```python
from build123d import *

# Parameters (mm, degrees)
EXTRUDE_1_DEPTH     = 24.5
FILLET_1_R          = 20
FILLET_2_R          = 9
SKETCH_2_W          = 18.5
SKETCH_2_H          = 26.060105981
CUT_EXTRUDE_1_DEPTH = 18
SKETCH_3_W          = 18.5
SKETCH_3_H          = 21.487076152
CUT_EXTRUDE_2_DEPTH = 18
FILLET_3_R          = 1
SKETCH_6_R          = 4
SKETCH_6_R_2        = 3.25
CUT_EXTRUDE_3_DEPTH = 129.841957452
SKETCH_7_R          = 6
CUT_EXTRUDE_4_DEPTH = 10
SKETCH_8_R          = 3.5
CUT_EXTRUDE_5_DEPTH = 127.09619344
EXTRUDE_START       = -10
SKETCH_9_R          = 4
SKETCH_9_R_2        = 3.5
EXTRUDE_2_DEPTH     = 10


with BuildPart() as part:
    # Эскиз1 → Бобышка-Вытянуть1 (new body)
    with BuildSketch(Plane.XY):
        Polygon((0, 0), (0, 40), (120, 40), (120, 0), (100, 0), (100, 29), (20, 29), (20, 0), align=None)
    extrude(amount=EXTRUDE_1_DEPTH)

    # Скругление1
    fillet_1_edges = [part.edges().sort_by_distance(p)[0] for p in [
        (0, 40, 12.25),
        (120, 40, 12.25),
    ]]
    fillet(fillet_1_edges, radius=FILLET_1_R)

    # Скругление2
    fillet_2_edges = [part.edges().sort_by_distance(p)[0] for p in [
        (100, 29, 12.25),
        (20, 29, 12.25),
    ]]
    fillet(fillet_2_edges, radius=FILLET_2_R)

    # Эскиз2 → Вырез-Вытянуть1 (cut)
    with BuildSketch(Plane(origin=(120, 0, 0), x_dir=(0, 0, -1), z_dir=(1, 0, 0))):
        with Locations((-12.25, 33.03005299)):
            Rectangle(SKETCH_2_W, SKETCH_2_H)
    extrude(amount=-CUT_EXTRUDE_1_DEPTH, mode=Mode.SUBTRACT)

    # Эскиз3 → Вырез-Вытянуть2 (cut)
    with BuildSketch(Plane.ZY):
        with Locations((12.25, 30.743538076)):
            Rectangle(SKETCH_3_W, SKETCH_3_H)
    extrude(amount=-CUT_EXTRUDE_2_DEPTH, mode=Mode.SUBTRACT)

    # Скругление3
    fillet_3_edges = [part.edges().sort_by_distance(p)[0] for p in [
        (20, 10, 0),
        (120, 10, 24.5),
        (0, 10, 0),
        (0, 10, 24.5),
        (60, 40, 0),
        (114.142135624, 34.142135624, 0),
        (5.857864376, 34.142135624, 0),
        (60, 40, 24.5),
        (114.142135624, 34.142135624, 24.5),
        (5.857864376, 34.142135624, 24.5),
        (60, 29, 0),
        (60, 29, 24.5),
        (100, 10, 0),
        (100, 10, 24.5),
        (22.636038969, 26.363961031, 0),
        (22.636038969, 26.363961031, 24.5),
        (97.363961031, 26.363961031, 0),
        (97.363961031, 26.363961031, 24.5),
        (20, 10, 24.5),
        (120, 10, 0),
    ]]
    fillet(fillet_3_edges, radius=FILLET_3_R)

    # Эскиз6 → Вырез-Вытянуть3 (cut, through all)
    with BuildSketch(Plane(origin=(0, 0, 0), x_dir=(-1, 0, 0), z_dir=(0, -1, 0))):
        with Locations(Location((-10, -12.25, 0), (0, 0, 180))):
            Circle(SKETCH_6_R)
        with Locations(Location((-110, -12.25, 0), (0, 0, 180))):
            Circle(SKETCH_6_R_2)
    extrude(amount=-CUT_EXTRUDE_3_DEPTH, mode=Mode.SUBTRACT)

    # Эскиз7 → Вырез-Вытянуть4 (cut)
    with BuildSketch(Plane(origin=(0, 20, 0), x_dir=(1, 0, 0), z_dir=(0, 1, 0))):
        with Locations(Location((10, -12.25, 0), (0, 0, 270))):
            Circle(SKETCH_7_R)
        with Locations(Location((110, -12.25, 0), (0, 0, 270))):
            Circle(SKETCH_7_R)
    extrude(amount=-CUT_EXTRUDE_4_DEPTH, mode=Mode.SUBTRACT)

    # Эскиз8 → Вырез-Вытянуть5 (cut, through all)
    with BuildSketch(Plane(origin=(0, 10, 0), x_dir=(1, 0, 0), z_dir=(0, 1, 0))):
        with Locations(Location((110, -12.25, 0), (0, 0, 270))):
            Circle(SKETCH_8_R)
    extrude(amount=-CUT_EXTRUDE_5_DEPTH, mode=Mode.SUBTRACT)

    # Эскиз9 → Бобышка-Вытянуть2 (add)
    with BuildSketch(Plane(origin=(0, 10, 0), x_dir=(1, 0, 0), z_dir=(0, 1, 0)).offset(EXTRUDE_START)):
        with Locations((10, -12.25)):
            Circle(SKETCH_9_R)
        with Locations(Location((10, -12.25, 0), (0, 0, 270))):
            Circle(SKETCH_9_R_2, mode=Mode.SUBTRACT)
    extrude(amount=EXTRUDE_2_DEPTH)


solid = part.part
```
For this review, take the finished solid that the model builds, in its own axes (mm). A direction names the side the tool comes from. Coordinates: 2 decimals unless noted, no trailing zeros. Loops run counter-clockwise (first coordinate to the right, second up) from the corner with the lowest first, then second, coordinate; pieces in that order, holes last. Notation, with made-up numbers: (69.5, 59.5) - (123.5, 59.5) arc R19 ccw to (123.5, 76.5) - close; hole circle Ø3 at (49, 82). An arc over 180 degrees is marked (long way). Use one line per item in the form item = value. Start each with the question number.
1) For faces 1 (the face through (112, 0, 9)), 2 (the face through (22.566, 26.294, 12.408)), 3 (the face through (11, 28, 21.5)), 4 (the face through (4.677, 15.07, 15.019)), 5 (the face through (6.583, 4.93, 11.491)), list the 3-axis set-ups (+Z, -Z, +X, -X, +Y, -Y) from which the entire face can be reached by the end or side of a thin tool; tool diameter is ignored.
2) Take a section at A-A (z = 12.25). State how many separate pieces and enclosed holes the cut face has, plus the area to 3 significant figures.
3) Draft analysis for pull direction X (two halves, no side actions). For faces 6 (the face through (13, 10, 15)), 7 (the face through (115, 20, 16)), 8 (the face through (18.184, 39.917, 10.636)), state which applies: released by +X, released by -X, zero draft, split by the parting line, or undercut.
4) Take a section at C-C (z = 7.5). State the section outline as (x, y) points, plus the area to 3 significant figures.
5) To check wall thickness, follow probe 1 along X at (y, z) = (15.5, 12.25); probe 2 along X at (y, z) = (2.5, 12.25); probe 3 along Z at (x, y) = (106, 21). State the ranges of each line that lie inside material, in increasing order. Write a range as from..to.
6) Take a section at B-B (x = 52.5). State the section outline as (y, z) points, plus the area to 3 significant figures.
7) For pin 1 (2 mm diameter, centred on y = 35.5, z = 5.5, fed in from +X); pin 2 (9 mm diameter, centred on x = 113.5, z = 8, fed in from +Y); pin 3 (3.5 mm diameter, centred on x = 111.5, z = 14, fed in from +Y); pin 4 (5.5 mm diameter, centred on x = 10, z = 12.25, fed in from -Y), all flat-tipped, find the tip position at first contact; note any pin that passes through.
From the geometry:
q1.face_1 = +Z, -Z, +X, -X, -Y
q1.face_2 = +Z, -Z, -Y
q1.face_3 = -X, +Y
q1.face_4 = +Y
q1.face_5 = +Y, -Y
q2.separate_pieces = 3
q2.enclosed_holes = 0
q2.area = 1,410 mm2
q3.face_6 = undercut
q3.face_7 = zero draft
q3.face_8 = released by -X
q4.outline = (0, 0) - (20, 0) - (20, 20) arc R9 cw to (29, 29) - (91, 29) arc R9 cw to (100, 20) - (100, 0) - (120, 0) - (120, 20) - (113.67, 20) - (113.67, 10) - (106.33, 10) - (106.33, 20) - (102, 20) - (102, 39.9) arc R20 ccw to (100, 40) - (20, 40) arc R20 ccw to (18, 39.9) - (18, 20) - (13.67, 20) - (13.67, 10) - (6.33, 10) - (6.33, 20) - (0, 20) - close
q4.area = 1,650 mm2
q5.probe_1 = 0..4, 16..20, 100..104, 116..120
q5.probe_2 = 0..6.5, 13.5..20, 100..106.5, 113.5..120
q5.probe_3 = 0..3, 21.5..24.5
q6.outline = (29, 1) arc R1 ccw to (30, 0) - (39, 0) arc R1 ccw to (40, 1) - (40, 23.5) arc R1 ccw to (39, 24.5) - (30, 24.5) arc R1 ccw to (29, 23.5) - close
q6.area = 269 mm2
q7.pin_1 = 102
q7.pin_2 = 20
q7.pin_3 = 10
q7.pin_4 = through
